from build123d import *

# Parameters (mm, degrees)
SKETCH1_W           = 72
SKETCH1_H           = 9
SKETCH1_R           = 1.25
SKETCH1_W_2         = 14
SKETCH1_H_2         = 2.8
SKETCH1_W_3         = 32
BOSS_EXTRUDE1_DEPTH = 0.15


with BuildPart() as part:
    # Sketch1 → Boss-Extrude1 (new body)
    with BuildSketch(Plane(origin=(0, 0, 0), x_dir=(1, 0, 0), z_dir=(0, 1, 0))):
        Rectangle(SKETCH1_W, SKETCH1_H)
        with Locations(Location((-18, 0, 0), (0, 0, 270))):
            Circle(SKETCH1_R, mode=Mode.SUBTRACT)
        with Locations(Location((18, 0, 0), (0, 0, 270))):
            Circle(SKETCH1_R, mode=Mode.SUBTRACT)
        with Locations((27, 0)):
            Rectangle(SKETCH1_W_2, SKETCH1_H_2, mode=Mode.SUBTRACT)
        Rectangle(SKETCH1_W_3, SKETCH1_H_2, mode=Mode.SUBTRACT)
        with Locations((-27, 0)):
            Rectangle(SKETCH1_W_2, SKETCH1_H_2, mode=Mode.SUBTRACT)
    extrude(amount=BOSS_EXTRUDE1_DEPTH)


solid = part.part
The listing builds one solid part. Answer for the finished solid, in the listing's coordinates (mm). Round coordinates to 2 decimals unless told otherwise and drop trailing zeros. Write each loop counter-clockwise with the first axis right and the second up, starting at its lowest first coordinate (ties: lowest second). Pieces come first, ordered by that corner, then holes. Notation, with made-up numbers: M -4,17.25 L 35,17.25 A30 cw 35,45.25 Z; hole C 35,69 d8. An arc over 180 degrees is marked long. Write each question's results on one line, items separated by ' | '. Start each with the question number.
Item 1: A cutting plane is placed at D-D on x = 28. Write down the section's boundary in (y, z), and give its area (3 significant figures).
Item 2: A cutting plane is placed at C-C on z = 0. Write down the section's boundary in (x, y), and give its area (3 significant figures).
Item 3: A cutting plane is placed at B-B on y = 0.05. Write down the section's boundary in (x, z).
Item 4: A cutting plane is placed at A-A on x = 18. Write down the section's boundary in (y, z).
Item 5: A flat-ended cylindrical pin translates along its axis: pin 1 Ø4 at (x, z) = (-18, 0) entering from +Y. Find the tip coordinate at first contact, or state that the pin passes through.
Item 6: Straight lines are drawn through the part: L1, parallel to X at y = 0.1, z = 0; L2, parallel to Z at x = -5.5, y = 0.05; L3, parallel to Z at x = -19, y = 0.1. For each, find the intervals that lie inside material, in ascending order. Write a range as [from, to].
Check sheet entries:
1) outline: M 0,-4.5 L 0.15,-4.5 L 0.15,-1.4 L 0,-1.4 Z; M 0,1.4 L 0.15,1.4 L 0.15,4.5 L 0,4.5 Z | area: 0.930 mm²
2) outline: M -36,0 L -34,0 L -34,0.15 L -36,0.15 Z; M -20,0 L -19.25,0 L -19.25,0.15 L -20,0.15 Z; M -16.75,0 L -16,0 L -16,0.15 L -16.75,0.15 Z; M 16,0 L 16.75,0 L 16.75,0.15 L 16,0.15 Z; M 19.25,0 L 20,0 L 20,0.15 L 19.25,0.15 Z; M 34,0 L 36,0 L 36,0.15 L 34,0.15 Z | area: 1.05 mm²
3) outline: M -36,-4.5 L 36,-4.5 L 36,4.5 L -36,4.5 Z; hole M -34,-1.4 L -20,-1.4 L -20,1.4 L -34,1.4 Z; hole C -18,0 d2.5; hole M -16,-1.4 L 16,-1.4 L 16,1.4 L -16,1.4 Z; hole C 18,0 d2.5; hole M 20,-1.4 L 34,-1.4 L 34,1.4 L 20,1.4 Z
4) outline: M 0,-4.5 L 0.15,-4.5 L 0.15,-1.25 L 0,-1.25 Z; M 0,1.25 L 0.15,1.25 L 0.15,4.5 L 0,4.5 Z
5) pin 1: y = 0.15
6) L1: [-36, -34], [-20, -19.25], [-16.75, -16], [16, 16.75], [19.25, 20], [34, 36] | L2: [-4.5, -1.4], [1.4, 4.5] | L3: [-4.5, -0.75], [0.75, 4.5]
